```python
from build123d import *

# Parameters (mm, degrees)
SALIENTE_EXTRUIR1_DEPTH = 10
CROQUIS2_R              = 25
SALIENTE_EXTRUIR3_DEPTH = 32
CROQUIS4_R              = 16
CORTAR_EXTRUIR1_DEPTH   = 15
CORTAR_EXTRUIR2_START   = -25.000000112
CORTAR_EXTRUIR2_DEPTH   = 50.000000224
NERVIO1_REACH           = 117.503
CROQUIS8_WALL_W         = 258.006455054
CROQUIS8_WALL_H         = 10
CROQUIS9_R              = 10
CROQUIS9_R_2            = 6.5
SALIENTE_EXTRUIR4_DEPTH = 6


# Read off the part's stored shape, not the designer's step: Cortar-Extruir2
with BuildPart() as part:
    # Croquis1 → Saliente-Extruir1 (new body)
    with BuildSketch(Plane(origin=(0, 0, 0), x_dir=(1, 0, 0), z_dir=(0, 1, 0))):
        with BuildLine():
            Line((-45.297427526, 18.379317433), (-23.745406297, 83.820209702))
            ThreePointArc((-23.745406297, 83.820209702), (0, 51), (23.745406297, 83.820209702))
            Line((23.745406297, 83.820209702), (45.297427526, 18.379317433))
            ThreePointArc((45.297427526, 18.379317433), (43.342628533, 5.793613586), (32, 0))
            Line((32, 0), (-32, 0))
            ThreePointArc((-32, 0), (-43.342628533, 5.793613586), (-45.297427526, 18.379317433))
        make_face()
    extrude(amount=SALIENTE_EXTRUIR1_DEPTH)

    # Croquis2 → Saliente-Extruir3 (add)
    with BuildSketch(Plane(origin=(0, 0, 0), x_dir=(1, 0, 0), z_dir=(0, 1, 0))):
        with Locations(Location((0, 76, 0), (0, 0, 161.771441232))):
            Circle(CROQUIS2_R)
    extrude(amount=SALIENTE_EXTRUIR3_DEPTH)

    # Croquis4 → Cortar-Extruir1 (cut)
    with BuildSketch(Plane(origin=(0, 32, 0), x_dir=(1, 0, 0), z_dir=(0, 1, 0))):
        with Locations(Location((0, 76, 0), (0, 0, 270))):
            Circle(CROQUIS4_R)
    extrude(amount=-CORTAR_EXTRUIR1_DEPTH, mode=Mode.SUBTRACT)

    # Cortar-Extruir2 outline → Cortar-Extruir2 (cut)
    with BuildSketch(Plane(origin=(0, 0, 0), x_dir=(0, 0, -1), z_dir=(1, 0, 0)).offset(CORTAR_EXTRUIR2_START)):
        with BuildLine():
            add(Edge.make_bspline(
                [(71, 24.5), (71, 25.830324865), (71.548602551, 27.119839879), (73.380983998, 28.951882233), (74.682846227, 29.499135225), (77.310580087, 29.500862615), (78.614537315, 28.956974901), (80.458235075, 27.112387922), (80.999440282, 25.812671971), (81.000558807, 23.191595456), (80.460035839, 21.889945603), (78.61477129, 20.042727881), (77.319144976, 19.500263352), (74.682852162, 19.499736848), (73.382124852, 20.047206111), (71.548344872, 21.880188876), (71, 23.169675135), (71, 24.5)],
                knots=[0, 0, 0, 0, 0.125, 0.125, 0.25, 0.25, 0.375, 0.375, 0.5, 0.5, 0.625, 0.625, 0.75, 0.75, 0.875, 0.875, 1, 1, 1, 1], degree=3))
        make_face()
    extrude(amount=CORTAR_EXTRUIR2_DEPTH, mode=Mode.SUBTRACT)

    # Croquis8 wall → Nervio1 (add, up to next)
    with BuildSketch(Plane(origin=(0, 17.5, -41.00002412), x_dir=(0, 0.600000926209, -0.799999305342), z_dir=(0, 0.799999305342, 0.600000926209)), mode=Mode.PRIVATE) as nervio1_sk1:
        Rectangle(CROQUIS8_WALL_W, CROQUIS8_WALL_H)
    nervio1_tool1 = extrude(nervio1_sk1.sketch, amount=-NERVIO1_REACH, mode=Mode.PRIVATE) - part.part
    add(nervio1_tool1.solids().sort_by_distance((0, 17.5, -41.00002412))[0])

    # Croquis9 → Saliente-Extruir4 (add)
    # profile 1 of 2: a face of its own
    with BuildSketch(Plane(origin=(0, 10, 0), x_dir=(1, 0, 0), z_dir=(0, 1, 0))):
        with Locations(Location((-32, 14, 0), (0, 0, 270))):
            Circle(CROQUIS9_R)
        with Locations(Location((-32, 14, 0), (0, 0, 270))):
            Circle(CROQUIS9_R_2, mode=Mode.SUBTRACT)
    # profile 2 of 2: a face of its own
    with BuildSketch(Plane(origin=(0, 10, 0), x_dir=(1, 0, 0), z_dir=(0, 1, 0))):
        with Locations(Location((32, 14, 0), (0, 0, 90))):
            Circle(CROQUIS9_R)
        with Locations(Location((32, 14, 0), (0, 0, 90))):
            Circle(CROQUIS9_R_2, mode=Mode.SUBTRACT)
    extrude(amount=SALIENTE_EXTRUIR4_DEPTH)


solid = part.part
```
Design review of the part built by this model. Coordinates are the model's own, in mm. A direction names the side the tool comes from. Round coordinates to 2 decimals unless told otherwise and drop trailing zeros. Write each loop counter-clockwise with the first axis right and the second up, starting at its lowest first coordinate (ties: lowest second). Pieces come first, ordered by that corner, then holes.
Item 1: For probe 1 along X at (y, z) = (12.05, -14); probe 2 along Z at (x, y) = (32, 14.15); probe 3 along Y at (x, z) = (-23, -75.5), list the stretches that pass through material, from the lowest coordinate up.
Item 2: We need section D-D on z = -76. State how many separate pieces and enclosed holes the cut face has, and give its area (3 significant figures).
Item 3: We need section C-C on y = 4.5. Write out the cut boundary in (x, z), and give its area (3 significant figures).
Item 4: We need section B-B on y = 12. Write out the cut boundary in (x, z), and give its area (3 significant figures).
Item 5: We need section A-A on z = -14. Write out the cut boundary in (x, y).
Item 6: Clearance check with flat-ended pins moving along their axes: pin 1 Ø5 at (y, z) = (9.5, -79.5) entering from +X; pin 2 Ø8 at (x, z) = (-32, -14) entering from +Y; pin 3 Ø4.5 at (y, z) = (18.5, -45.5) entering from -X; pin 4 Ø4 at (x, z) = (-11.5, -42) entering from -Y. State where each tip first meets the part, or that it passes through.
Item 7: The part is to be moulded in two halves that separate along Z. For faces 1 (the flat face through (-0.07, 17.58, -41.11)), 2 (the cylindrical face through (-25.555, 12.958, -14.846)), 3 (the flat face through (39, 16, -14)), say which applies: +Z half, -Z half, draft (parallel to the pull), parting line (faces both ways), or undercut.
Item 8: For faces 4 (the flat face through (-5, 15, -43)), 5 (the cylindrical face through (43.45, 4.93, -5.944)), 6 (the flat face through (-16, 32, -81)), 7 (the cylindrical face through (25.555, 12.958, -13.154)), 8 (the flat face through (5, 15, -43)), list the 3-axis set-ups (+Z, -Z, +X, -X, +Y, -Y) from which the entire face can be reached by the end or side of a thin tool; tool diameter is ignored.
Returned:
1. probe 1: x = -42 to -38.5, -25.5 to -22, 22 to 25.5, 38.5 to 42
1. probe 2: z = -24 to -20.5, -7.5 to -4
1. probe 3: y = 0 to 19.53, 29.47 to 32
2. separate pieces: 3
2. enclosed holes: 0
2. area: 966 mm2
3. outline: (-45.3, -18.38) - (-23.75, -83.82) arc R25 ccw to (23.75, -83.82) - (45.3, -18.38) arc R14 ccw to (32, 0) - (-32, 0) arc R14 ccw to start
3. area: 6,720 mm2
4. outline: circle Ø20 at (-32, -14); (-5, -51.51) arc R25 ccw (long way) to (5, -51.51) - (5, -33.67) - (-5, -33.67) - close; circle Ø20 at (32, -14); hole circle Ø13 at (-32, -14); hole circle Ø13 at (32, -14)
4. area: 2,500 mm2
5. outline: (-46, 0) - (46, 0) - (46, 10) - (42, 10) - (42, 16) - (38.5, 16) - (38.5, 10) - (25.5, 10) - (25.5, 16) - (22, 16) - (22, 10) - (-22, 10) - (-22, 16) - (-25.5, 16) - (-25.5, 10) - (-38.5, 10) - (-38.5, 16) - (-42, 16) - (-42, 10) - (-46, 10) - close
6. pin 1: stops at x = 25.99
6. pin 2: stops at y = 10
6. pin 3: stops at x = -5
6. pin 4: stops at y = 0
7. face 1: +Z half
7. face 2: undercut
7. face 3: draft
8. face 4: +Z, -X, +Y
8. face 5: +X, +Y, -Y
8. face 6: +Z, -Z, +X, -X, +Y
8. face 7: +Y
8. face 8: +Z, +X, +Y
